Build history of the part. All positions in model axes, mm. Face numbers are marked on the shaded views. A direction names the side the tool comes from. Coordinates: 2 decimals unless noted, no trailing zeros. Order: outer loops, then holes, each group sorted by start corner. A loop starts at its lowest first (then second) coordinate and runs counter-clockwise, first axis right, second up. Notation, with made-up numbers: (89.5, 45) - (129.5, 45) arc R27 ccw to (129.5, 61) - close; hole circle Ø5 at (63, -0.75). An arc over 180 degrees is marked (long way). Return JSON: item names as keys, results as strings.
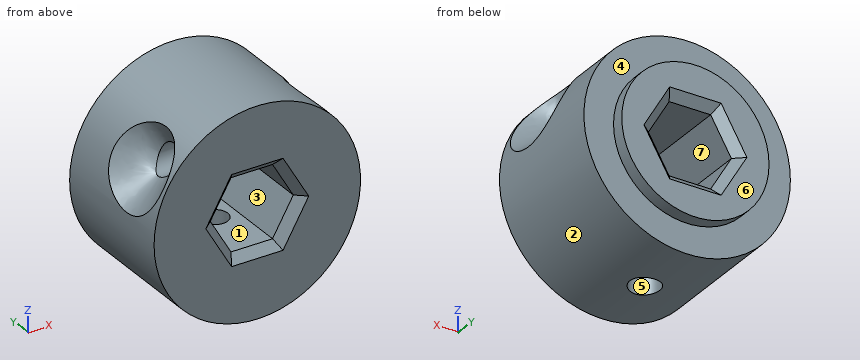
Autodesk Inventor part; units mm, degrees
ref_plane "Work Plane2" through (0, 0, -19.05) normal (0, 0, 1) x (1, 0, 0)
ref_plane "YZ Plane" through (0, 0, 0) normal (1, 0, 0) x (0, 1, 0)
ref_plane "XZ Plane" through (0, 0, 0) normal (0, 1, 0) x (-1, 0, 0)
sketch "Sketch9" plane through (0, 0, 0) normal (0, 1, 0) x (-1, 0, 0)
  circle A0 centre (0, 0) radius 19.05
  dimension "d53" = 38.1
extrude "Extrusion6" add sketch "Sketch9" along normal mid plane 24.257
sketch "Sketch10" plane through (0, 12.1285, 0) normal (0, 1, 0) x (1, 0, 0)
  circle A0 centre (0, 0) radius 13.589
  dimension "idWasher" = 27.178
extrude "Extrusion7" add sketch "Sketch10" along normal blind 2.3707
sketch "Sketch11" plane through (0, 14.4992, 0) normal (0, 1, 0) x (1, 0, 0)
  line L0 (7.6623, 0) -> (3.8312, -6.6358)
  line L1 (3.8312, -6.6358) -> (-3.8312, -6.6358)
  line L2 (-3.8312, -6.6358) -> (-7.6623, 0)
  line L3 (-7.6623, 0) -> (-3.8312, 6.6357)
  line L4 (-3.8312, 6.6357) -> (3.8312, 6.6357)
  line L5 (3.8312, 6.6357) -> (7.6623, 0)
  point P0 (0, 0)
  point P1 (0, 0)
  dimension "d59" = 13.2715
extrude "Extrusion8" cut sketch "Sketch11" against normal through all
sketch "Sketch12" plane through (0, 0, 0) normal (1, 0, 0) x (0, 1, 0)
  circle A0 centre (-4.0428, 9.1758) radius 2.54
  line L0 (14.4992, 0) -> (-12.1285, 0)
  line L1 (-12.1285, 19.05) -> (-12.1285, -19.05)
  point P0 (0, 0)
  dimension "d62" = 5.08
  dimension "d63" = 9.1758
  dimension "oneThirdSpoolHeight" = 8.0857
extrude "Extrusion9" cut sketch "Sketch12" along normal through all both and the other way through all
chamfer "Chamfer5" distance 4.7625 angle 45 2 edges at (16.6229, -6.5796, 9.3048) (-16.6229, -6.5796, 9.3048)
ref_plane "Work Plane2" through (0, 0, -19.05) normal (0, 0, 1) x (1, 0, 0)
sketch "Sketch13" plane through (0, 0, -19.05) normal (0, 0, 1) x (1, 0, 0)
  point P0 (0, 0)
  point P1 (0, 0)
hole "Hole2" at (0, 0, -19.05) direction (0, 0, 1) diameter 4.699 depth 12.4143 counterbore diameter 5.5372 counterbore depth 5.5626
chamfer "Chamfer6" distance 1.5875 angle 45 12 edges at (-5.7467, 14.4992, -3.3179) (0, 14.4992, -6.6357) (5.7467, 14.4992, -3.3179) (5.7467, 14.4992, 3.3179) (0, 14.4992, 6.6358) (-5.7467, 14.4992, 3.3179) (0, -12.1285, 6.6358) (5.7467, -12.1285, 3.3179) (5.7467, -12.1285, -3.3179) (0, -12.1285, -6.6357) (-5.7467, -12.1285, -3.3179) (-5.7467, -12.1285, 3.3179)
equation "\"d53\" = spoolInteriorDiameter"
equation "\"d59\" = hexDiameter"
equation "\"d62\" = holeForString"
equation "\"d63\" = stringHoleCenterFromHexShaft"
equation "\"oneThirdSpoolHeight\" = 0.333333 * singleSpoolHeight"
equation "\"d67\" = stringHoleChamfer"
equation "\"d77\" = hexHoleChamfer"
equation "\"holeForString\" = stringDiameter + clearanceForString"
equation "\"stringDiameter\" = 3.048"
equation "\"clearanceForString\" = 2.032"
equation "\"spoolHeightWithoutSpacer\" = 69.85"
equation "\"hexShaftDiameter\" = 12.7"
equation "\"clearanceForHexShaft\" = 0.5715"
equation "\"hexDiameter\" = hexShaftDiameter + clearanceForHexShaft"
equation "\"supportChannels\" = 3.81"
equation "\"spoolInteriorDiameter\" = 38.1"
equation "\"spoolInteriroRadius\" = 0.5 * spoolInteriorDiameter"
equation "\"spoolExteriorDiameter\" = 88.9"
equation "\"spoolExteriorRadius\" = 0.5 * spoolExteriorDiameter"
equation "\"spoolFiletRadius\" = 0.5 * supportChannels"
equation "\"holeCenter\" = 0.25 * spoolHeightWithoutSpacer - 0.75 * supportChannels"
equation "\"hexHoleChamfer\" = 1.5875"
equation "\"stringHoleCenterFromHexShaft\" = 0.5 * hexDiameter + 0.5 * holeForString"
equation "\"textCircleDiameter\" = 0.75 * spoolExteriorDiameter"
equation "\"textHeight\" = 6.096"
equation "\"textDepth\" = 1.27"
equation "\"stringHoleChamfer\" = 4.7625"
equation "\"spoolTotalHeight\" = 76.2"
equation "\"spaceHeight\" = spoolTotalHeight - spoolHeightWithoutSpacer"
equation "\"spacerDiameter\" = 24.13"
properties part number "spoolV04" material "PC/ABS Plastic"
1. Cut at C-C on z = -3.5. Give the cut face in (x, y).
Check values:
{"outline": "(-18.73, -12.13) - (-7.47, -12.13) - (-5.64, -10.54) - (-5.64, 12.91) - (-7.47, 14.5) - (-13.13, 14.5) - (-13.13, 12.13) - (-18.73, 12.13) - close; (5.64, -10.54) - (7.47, -12.13) - (18.73, -12.13) - (18.73, 12.13) - (13.13, 12.13) - (13.13, 14.5) - (7.47, 14.5) - (5.64, 12.91) - close"}
2. Tool access for the marked faces 5, 6 and 7: list every direction of +Z, -Z, +X, -X, +Y, -Y with a clear straight run to the whole face (end or side of a thin tool).
Check values:
{"face 5": "-Z", "face 6": "+Z, -Z, +X, -X, +Y", "face 7": "+Y, -Y"}
3. Cut at A-A on y = 7. Give the cut face in (x, z).
Check values:
{"outline": "circle Ø38.1 at (0, 0); hole (-7.66, 0) - (-3.83, -6.64) - (3.83, -6.64) - (7.66, 0) - (3.83, 6.64) - (-3.83, 6.64) - close"}
4. Probe L1, parallel to Z at x = 0, y = 7.75; L2, parallel to Z at x = -2, y = 2.25; L3, parallel to X at y = 0, z = -16.1. List the from-to ranges inside material, lowest first.
Check values:
{"L1": "-19.05 to -6.64, 6.64 to 19.05", "L2": "-18.94 to -6.64, 6.64 to 18.94", "L3": "-10.18 to -2.77, 2.77 to 10.18"}
5. Cut at B-B on x = 0. Give the cut face in (y, z).
Check values:
{"outline": "(-12.13, -19.05) - (-2.77, -19.05) - (-2.77, -13.49) - (-2.35, -13.49) - (-2.35, -6.64) - (-10.54, -6.64) - (-12.13, -8.22) - close; (-12.13, 8.22) - (-10.54, 6.64) - (12.91, 6.64) - (14.5, 8.22) - (14.5, 13.59) - (12.13, 13.59) - (12.13, 19.05) - (-12.13, 19.05) - close; (2.35, -13.49) - (2.77, -13.49) - (2.77, -19.05) - (12.13, -19.05) - (12.13, -13.59) - (14.5, -13.59) - (14.5, -8.22) - (12.91, -6.64) - (2.35, -6.64) - close; hole circle Ø5.08 at (-4.04, 9.18)"}
6. Mould opens along Z. For the marked faces 1, 2, 3 and 4 say: pulls with the +Z half, pulls with the -Z half, needs draft (parallel to the pull), parting line crosses it, or undercut.
Check values:
{"face 1": "undercut", "face 2": "parting line crosses it", "face 3": "undercut", "face 4": "needs draft"}
7. Drop flat-ended pins along their axis: pin 1 (4 mm diameter, centred on x = -1.5, y = -3, fed in from +Z); pin 2 (4 mm diameter, centred on x = 1.5, y = 0, fed in from -Z); pin 3 (5 mm diameter, centred on x = 12, y = 5, fed in from +Z); pin 4 (4.5 mm diameter, centred on y = -4.04, z = 9.18, fed in from -X). Give the stop position or say it passes through.
Check values:
{"pin 1": "z = 19.05", "pin 2": "z = -18.95", "pin 3": "z = 16.51", "pin 4": "through"}
